Design review of the part built by this model. Coordinates are the model's own, in mm. Face numbers are marked on the shaded views. A direction names the side the tool comes from. Coordinates: 2 decimals unless noted, no trailing zeros. Loops run counter-clockwise (first coordinate to the right, second up) from the corner with the lowest first, then second, coordinate; pieces in that order, holes last. Notation, with made-up numbers: (-10, -24.5) -> (32, -24.5) arc R26 ccw to (32, 4.5) -> close; hole circle Ø4 at (48, 26.25). An arc over 180 degrees is marked (long way). Answer as a JSON object with one key per item and string values.
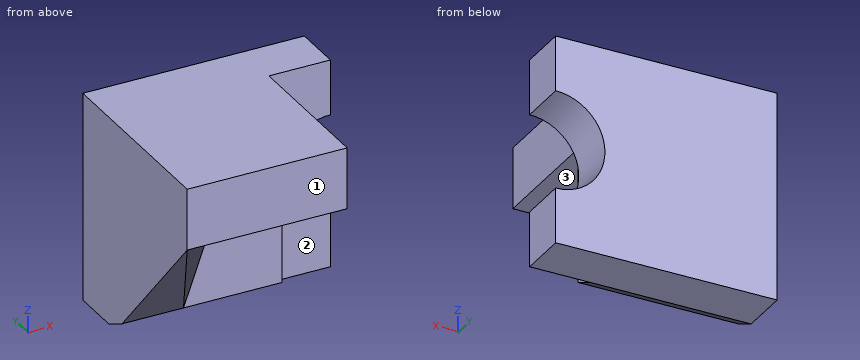
```python
from build123d import *

# Parameters (mm, degrees)
F0_W     = 90
F0_H     = 85
F1_DEPTH = 20
F3_DEPTH = 25
F6_DEPTH = 65


with BuildPart() as f1:
    # F0 (on Front) → F1 (new body)
    with BuildSketch(Plane.XZ):
        Rectangle(F0_W, F0_H)
    extrude(amount=F1_DEPTH)

    # F2 (on Front) → F3 (cut)
    with BuildSketch(Plane.XZ):
        with BuildLine():
            Line((45, -20), (45, 20))
            ThreePointArc((45, 20), (25, 0), (45, -20))
        make_face()
    extrude(amount=F3_DEPTH, mode=Mode.SUBTRACT)

    # F5 (on offset) → F6 (join)
    with BuildSketch(Plane.YZ.offset(20)):
        Polygon((-20, 20), (-20, 42.5), (-80, 42.5), (-80, 17.5), (-30, 17.5), (-30, -37.5), (-20, -42.5), (-20, -20), align=None)
    extrude(amount=-F6_DEPTH)

    # F8 (on face) → F10 section 0
    with BuildSketch(Plane.XZ.offset(30), mode=Mode.PRIVATE) as f10_s0:
        Polygon((-45, -37.5), (-20, -37.5), (0, 17.5), (-45, 17.5), align=None)
    loft([f10_s0.sketch, Vertex(-45, -80, 17.5)])


solid = f1.part
```
1) Wall thickness on probe 1 along Y at (x, z) = (-1, -14.5); probe 2 along Z at (x, y) = (-7, -54); probe 3 along X at (y, z) = (-21.5, 4.5): over which ranges is each line inside the solid? List them lowest first.
Completed:
{"probe 1": "-30 to 0", "probe 2": "17.5 to 42.5", "probe 3": "-45 to 20"}
2) Add section B-B, the plane x = 8. Give the boundary of the cut face in (y, z).
Completed:
{"outline": "(-80, 17.5) -> (-30, 17.5) -> (-30, -37.5) -> (-20, -42.5) -> (0, -42.5) -> (0, 42.5) -> (-80, 42.5) -> close"}
3) Add section D-D, the plane x = -27. Give the boundary of the cut face in (y, z).
Completed:
{"outline": "(-80, 17.5) -> (-60, 17.5) -> (-44, -22.1) -> (-30, -37.5) -> (-20, -42.5) -> (0, -42.5) -> (0, 42.5) -> (-80, 42.5) -> close"}
4) For the marked faces 1, 2 and 3, list the 3-axis set-ups (+Z, -Z, +X, -X, +Y, -Y) from which the entire face can be reached by the end or side of a thin tool; tool diameter is ignored.
Completed:
{"face 1": "+Z, -Z, +X, -X, -Y", "face 2": "+Z, -Z, +X, -Y", "face 3": "-Z, +X, -Y"}
5) Clearance check with flat-ended pins moving along their axes: pin 1 Ø5 at (x, z) = (2.5, -5.5) entering from +Y; pin 2 Ø18 at (y, z) = (-39.5, 10.5) entering from +X; pin 3 Ø15 at (x, y) = (-9.5, -53) entering from -Z; pin 4 Ø5 at (y, z) = (-13.5, 1.5) entering from +X. State where each tip first meets the part, or that it passes through.
Completed:
{"pin 1": "y = 0", "pin 2": "x = 20", "pin 3": "z = 17.5", "pin 4": "x = 25.4"}
6) Add section C-C, the plane y = -33. Give the boundary of the cut face in (x, z).
Completed:
{"outline": "(-45, -34.2) -> (-21.5, -34.2) -> (-2.7, 17.5) -> (20, 17.5) -> (20, 42.5) -> (-45, 42.5) -> close"}
7) Add section A-A, the plane z = 12. Give the boundary of the cut face in (x, y), and give its area (3 significant figures).
Completed:
{"outline": "(-45, -75) -> (-42.5, -75) -> (-2, -30) -> (20, -30) -> (20, -20) -> (29, -20) -> (29, 0) -> (-45, 0) -> close", "area": "3,150 mm²"}
